Geometry check sheet. Reference: the model listing, model coordinates, mm. Coordinates: 2 decimals unless noted, no trailing zeros. Loops run counter-clockwise (first coordinate to the right, second up) from the corner with the lowest first, then second, coordinate; pieces in that order, holes last. Notation, with made-up numbers: (41.5, -39.75) - (75.5, -39.75) arc R29 cw to (75.5, -12.75) - close; hole circle Ø5 at (74, 39.5). An arc over 180 degrees is marked (long way). Write item = value, one per line. Start each with the question number.
from build123d import *

# Parameters (mm, degrees)
F0_W     = 101.4645919204
F0_H     = 97.2314924002
F1_DEPTH = 25.4
F3_DEPTH = 50.8
F5_DEPTH = 97.2324925002


with BuildPart() as f1:
    # F0 (on Top) → F1 (new body)
    with BuildSketch(Plane.XY):
        Rectangle(F0_W, F0_H)
    extrude(amount=F1_DEPTH)

    # F2 (on Top) → F3 (join)
    with BuildSketch(Plane.XY):
        with BuildLine():
            add(Edge.make_bspline(
                [(26.9378982484, -7.8889131546), (36.1832899021, 23.6808880022), (-8.8462532974, 19.7293571557), (-53.8757964969, 15.7778263092), (-18.0916449511, -11.8404440011), (17.6925065947, -39.4587143115), (26.9378982484, -7.8889131546)],
                knots=[0, 0, 0, 2.0943951024, 2.0943951024, 4.1887902048, 4.1887902048, 6.2831853072, 6.2831853072, 6.2831853072], degree=2, weights=[1, 0.5, 1, 0.5, 1, 0.5, 1]))
        make_face()
    extrude(amount=F3_DEPTH)

    # F4 (on face) → F5 (cut, through all)
    with BuildSketch(Plane.XZ.offset(48.6157462001)):
        Polygon((27.4616602615, 50.8), (-27.4616602615, 50.8), (27.4616602615, 25.4), align=None)
    extrude(amount=-F5_DEPTH, mode=Mode.SUBTRACT)


solid = f1.part
(1) Depth check by flat-ended pin: pin 1 (2 mm diameter, centred on x = -4.5, y = 0.5, fed in from +Z); pin 2 (2 mm diameter, centred on x = 34, y = -0.5, fed in from +Z); pin 3 (6 mm diameter, centred on x = -33, y = -4.5, fed in from -Z). Enter the tip coordinate at first touch or a pass-through.
(2) Sectioned sample at B-B on x = 41.5. Enter the section's corners in (y, z), plus the area to 3 significant figures.
(3) Scan lines: line 1 (Z direction, x = 0.5, y = -43); line 2 (Z direction, x = 18, y = 9.5); line 3 (Y direction, x = 8, z = 28.5). Record each from-to range of solid material in increasing order.
(4) Sectioned sample at A-A on y = -29.5. Enter the section's corners in (x, z).
(5) Draft check along X on faces 1 (the face through (-50.732, -1, 13)), 2 (the face through (-1, -48.616, 13)), 3 (the face through (50.732, -1, 13)). Enter one of: pulls with the +X half, pulls with the -X half, needs draft (parallel to the pull), parting line crosses it, or undercut.
Working result:
q1.pin_1 = 40.64
q1.pin_2 = 25.4
q1.pin_3 = 0
q2.outline = (-48.62, 0) - (48.62, 0) - (48.62, 25.4) - (-48.62, 25.4) - close
q2.area = 2,470 mm2
q3.line_1 = 0 to 25.4
q3.line_2 = 0 to 29.78
q3.line_3 = -19.79 to 17.35
q4.outline = (-50.73, 0) - (50.73, 0) - (50.73, 25.4) - (-50.73, 25.4) - close
q5.face_1 = pulls with the -X half
q5.face_2 = needs draft
q5.face_3 = pulls with the +X half
